Check sheet for the modelled part. Datum: model origin and axes. Units: mm. A direction names the side the tool comes from. Give positions to 0.01 mm unless a question says otherwise; leave off trailing zeros. Write each loop counter-clockwise with the first axis right and the second up, starting at its lowest first coordinate (ties: lowest second). Pieces come first, ordered by that corner, then holes. Notation, with made-up numbers: (80, 55.5) -> (116, 55.5) arc R24 ccw to (116, 68.5) -> close; hole circle Ø10 at (-22.5, -1). An arc over 180 degrees is marked (long way). Use a Markdown table: item, result. Add a question column.
1. Cross-section at C-C (x = -6.35). Enter the section's corners in (y, z), then the cut area to 3 significant figures.
2. Gauge pin test, flat ends, axial feed: P1, Ø1.5, axis at x = -110.5, z = -29, coming from the +Y side; P2, Ø2.5, axis at y = 68.5, z = -46, coming from the +X side; P3, Ø12, axis at y = 56.5, z = -9.5, coming from the -X side; P4, Ø7, axis at x = -158.75, z = -82.55, coming from the +Y side. Record the tip position at first contact, or that the pin passes through.
3. Cross-section at D-D (z = -34). Enter the section's corners in (x, y).
4. Scan lines: probe 1 along X at (y, z) = (4.25, -6.35); probe 2 along X at (y, z) = (4, -82); probe 3 along Z at (x, y) = (-96, 27.5). Record each from-to range of solid material in increasing order. Write a range as [from, to].
5. Cross-section at A-A (x = -144). Enter the section's corners in (y, z).
6. Release check for a two-part mould opening along Z. For faces 1 (the flat face through (-81, 35, -88.9)), 2 (the cylindrical face through (-4.3, 3.13, -85.76)), 3 (the flat face through (0, 3, -44)) record: released by +Z, released by -Z, zero draft, split by the parting line, or undercut.
7. Set-up check for faces 4 (the flat face through (-159, 6.35, -45)), 5 (the flat face through (-6, 6.35, -45)), 6 (the flat face through (-139.7, 25, -44)): record each of +Z, -Z, +X, -X, +Y, -Y from which the full face is reachable in a straight line by a thin tool's end or side.
8. Cross-section at B-B (y = 31.5). Enter the section's corners in (x, z), then the cut area to 3 significant figures.
from build123d import *

# Parameters (mm, degrees)
SKETCH1_W           = 165.1
SKETCH1_H           = 88.9
SKETCH1_R           = 3.81
BOSS_EXTRUDE1_DEPTH = 6.35
SKETCH2_W           = 139.7
SKETCH2_H           = 88.9
BOSS_EXTRUDE2_DEPTH = 57.15
SKETCH3_W           = 114.3
SKETCH3_H           = 63.5
CUT_EXTRUDE1_DEPTH  = 50.8
BOSS_EXTRUDE3_DEPTH = 2.54
BOSS_EXTRUDE4_DEPTH = 5.08


with BuildPart() as part:
    # Sketch1 → Boss-Extrude1 (new body)
    with BuildSketch(Plane(origin=(0, 0, 0), x_dir=(1, 0, 0), z_dir=(0, 1, 0))):
        with Locations((-82.55, 44.45)):
            Rectangle(SKETCH1_W, SKETCH1_H)
        with Locations((-158.75, 6.35)):
            Circle(SKETCH1_R, mode=Mode.SUBTRACT)
        with Locations((-158.75, 82.55)):
            Circle(SKETCH1_R, mode=Mode.SUBTRACT)
        with Locations((-6.35, 82.55)):
            Circle(SKETCH1_R, mode=Mode.SUBTRACT)
        with Locations((-6.35, 6.35)):
            Circle(SKETCH1_R, mode=Mode.SUBTRACT)
    extrude(amount=BOSS_EXTRUDE1_DEPTH)

    # Sketch2 → Boss-Extrude2 (add)
    with BuildSketch(Plane(origin=(0, 6.35, 0), x_dir=(1, 0, 0), z_dir=(0, 1, 0))):
        with Locations((-82.55, 44.45)):
            Rectangle(SKETCH2_W, SKETCH2_H)
    extrude(amount=BOSS_EXTRUDE2_DEPTH)

    # Sketch3 → Cut-Extrude1 (cut)
    with BuildSketch(Plane(origin=(0, 0, 0), x_dir=(-1, 0, 0), z_dir=(0, -1, 0))):
        with Locations((82.55, 44.45)):
            Rectangle(SKETCH3_W, SKETCH3_H)
    extrude(amount=-CUT_EXTRUDE1_DEPTH, mode=Mode.SUBTRACT)

    # Sketch5 → Boss-Extrude3 (add)
    with BuildSketch(Plane(origin=(0, 63.5, 0), x_dir=(1, 0, 0), z_dir=(0, 1, 0))):
        Polygon((-152.4, 88.9), (-152.4, 0), (-12.7, 0), (-12.7, 5.08), (-147.32, 5.08), (-147.32, 83.82), (-12.7, 83.82), (-12.7, 88.9), align=None)
    extrude(amount=BOSS_EXTRUDE3_DEPTH)

    # Sketch6 → Boss-Extrude4 (add)
    with BuildSketch(Plane(origin=(0, 66.04, 0), x_dir=(1, 0, 0), z_dir=(0, 1, 0))):
        Polygon((-147.32, 5.08), (-12.7, 5.08), (-12.7, 10.16), (-142.24, 10.16), (-142.24, 78.74), (-12.7, 78.74), (-12.7, 83.82), (-147.32, 83.82), align=None)
        Polygon((-12.7, 5.08), (-147.32, 5.08), (-147.32, 83.82), (-12.7, 83.82), (-12.7, 88.9), (-152.4, 88.9), (-152.4, 0), (-12.7, 0), align=None)
    extrude(amount=BOSS_EXTRUDE4_DEPTH)


solid = part.part
Worked answers:
| question | item | result |
|---|---|---|
| 1 | outline | (0, -88.9) -> (6.35, -88.9) -> (6.35, -86.36) -> (0, -86.36) -> close; (0, -78.74) -> (6.35, -78.74) -> (6.35, -10.16) -> (0, -10.16) -> close; (0, -2.54) -> (6.35, -2.54) -> (6.35, 0) -> (0, 0) -> close |
| 1 | area | 468 mm² |
| 2 | P1 | stops at y = 63.5 |
| 2 | P2 | stops at x = -142.24 |
| 2 | P3 | stops at x = -152.4 |
| 2 | P4 | passes through |
| 3 | outline | (-165.1, 0) -> (-139.7, 0) -> (-139.7, 50.8) -> (-25.4, 50.8) -> (-25.4, 0) -> (0, 0) -> (0, 6.35) -> (-12.7, 6.35) -> (-12.7, 63.5) -> (-147.32, 63.5) -> (-147.32, 66.04) -> (-142.24, 66.04) -> (-142.24, 71.12) -> (-152.4, 71.12) -> (-152.4, 6.35) -> (-165.1, 6.35) -> close |
| 4 | probe 1 | x = [-165.1, -162.56], [-154.94, -10.16], [-2.54, 0] |
| 4 | probe 2 | x = [-165.1, -162.52], [-154.98, -10.12], [-2.58, 0] |
| 4 | probe 3 | z = [-88.9, -76.2], [-12.7, 0] |
| 5 | outline | (0, -88.9) -> (71.12, -88.9) -> (71.12, 0) -> (0, 0) -> close; hole (63.5, -83.82) -> (66.04, -83.82) -> (66.04, -5.08) -> (63.5, -5.08) -> close |
| 6 | face 1 | released by -Z |
| 6 | face 2 | undercut |
| 6 | face 3 | zero draft |
| 7 | face 4 | +Z, -Z, -X, +Y |
| 7 | face 5 | +Z, -Z, +X, +Y |
| 7 | face 6 | -Y |
| 8 | outline | (-152.4, -88.9) -> (-12.7, -88.9) -> (-12.7, 0) -> (-152.4, 0) -> close; hole (-139.7, -76.2) -> (-25.4, -76.2) -> (-25.4, -12.7) -> (-139.7, -12.7) -> close |
| 8 | area | 5,160 mm² |
